Geometry check sheet. Reference: the model listing, model coordinates, mm. A direction names the side the tool comes from. Round coordinates to 2 decimals unless told otherwise and drop trailing zeros. Order: outer loops, then holes, each group sorted by start corner. A loop starts at its lowest first (then second) coordinate and runs counter-clockwise, first axis right, second up. Notation, with made-up numbers: (74, 72.5) - (101, 72.5) arc R15 cw to (101, 83.5) - close; hole circle Ø10 at (-19, 36). An arc over 180 degrees is marked (long way). One line per question, with ' | ' between items. Start each with the question number.
Q1. Gauge pin test, flat ends, axial feed: P1, Ø5, axis at x = 1016, z = 9.5, coming from the -Y side; P2, Ø5.5, axis at x = 620.64, y = 525.38, coming from the +Z side; P3, Ø2, axis at y = -198.5, z = 8.5, coming from the -X side; P4, Ø1, axis at x = 1180.5, z = 14, coming from the -Y side. Record the tip position at first contact, or that the pin passes through.
Q2. Sectioned sample at A-A, the plane x = 1039.5. Enter the section's corners in (y, z) (3 decimals), then the cut area to 3 significant figures.
Q3. Mould release check, pull along Y, two halves, no side actions. Record for faces 1 (the face through (1024.915, 215.072, 9.392)), 2 (the face through (916.535, 592.185, 9.392)), 3 (the face through (653.954, 499.757, 9.392)): +Y half, -Y half, draft (parallel to the pull), parting line (faces both ways), or undercut.
Q4. Material ranges on line 1 along Y through (x, z) = (1060, 1.75); line 2 along Y through (x, z) = (1069.5, 7.75); line 3 along X through (y, z) = (219, 13.75), recorded low to high.
Q5. Sectioned sample at C-C, the plane z = 4. Give the number of separate pieces and of enclosed holes in the cut face, then the cut area to 3 significant figures.
Q6. Tool access check on faces 4 (the face through (960.42, 143.22, 9.39)), 5 (the face through (982.65, -163.13, 9.39)), 6 (the face through (989.135, -122.216, 4.696)). Record the directions out of +Z, -Z, +X, -X, +Y, -Y that give a thin tool (end or side, any length) a straight path to the whole face; none if there is none.
Q7. Sectioned sample at B-B, the plane y = -16. Enter the section's corners in (x, z), then the cut area to 3 significant figures.
```python
from build123d import *

# Parameters (mm, degrees)
F1_DEPTH = 19.05
F3_DEPTH = 9.525
F5_DEPTH = 9.525
F6_W     = 94.742
F6_H     = 19.05
F6_H_2   = 22.0252738774
F7_DEPTH = 19.558
F8_R     = 3.302
F9_DEPTH = 19.051


# Not quite as in the source:
# - ends of sketch curves that miss each other by under 0.0002 mm in the source are joined
# - a feature names something its author has since deleted; it is built from what else it names
# - the program builds the solid bodies; features that only make, move or delete a surface that nothing else refers to are left out


with BuildPart() as f1:
    # F0 (on Top) → F1 (new body)
    with BuildSketch(Plane.XY):
        with BuildLine():
            Line((727.2677384075, 507.6293858847), (727.2677384075, -289.3185215378))
            ThreePointArc((727.2677384075, -289.3185215378), (771.8616098047, -333.912392935), (816.4554812019, -289.3185215378))
            Line((816.4554812019, -289.3185215378), (816.4554812019, -221.6290421598))
            Line((816.4554812019, -221.6290421598), (1153.5588304871, -102.9697649078))
            Line((1153.5588304871, -102.9697649078), (1192.9737952894, -152.2336658633))
            ThreePointArc((1192.9737952894, -152.2336658633), (1256.5580507142, -165.3785793409), (1281.2649482254, -105.3342998163))
            Line((1281.2649482254, -105.3342998163), (881.6774022659, 394.10141923))
            ThreePointArc((881.6774022659, 394.10141923), (879.6100790274, 397.83144491), (878.8940586752, 402.0355181492))
            Line((878.8940586752, 402.0355181492), (878.8940586752, 569.9420720746))
            ThreePointArc((878.8940586752, 569.9420720746), (881.2296299338, 577.2815963686), (887.3773054254, 581.9215959395))
            Line((887.3773054254, 581.9215959395), (946.5202680448, 602.7397254948))
            Line((946.5202680448, 602.7397254948), (904.3527355464, 722.5349641439))
            Line((904.3527355464, 722.5349641439), (884.020881133, 715.3782178375))
            Line((884.020881133, 715.3782178375), (880.8583161956, 724.3628607361))
            Line((880.8583161956, 724.3628607361), (549.7442765695, 607.8118009104))
            Line((549.7442765695, 607.8118009104), (552.906841507, 598.8271580117))
            Line((552.906841507, 598.8271580117), (544.9670195991, 596.0323666485))
            Line((544.9670195991, 596.0323666485), (582.9177988478, 488.2166518643))
            ThreePointArc((582.9177988478, 488.2166518643), (589.40821497, 480.9809077363), (599.1140759625, 480.4538812492))
            Line((599.1140759625, 480.4538812492), (710.3509851577, 519.6089097496))
            ThreePointArc((710.3509851577, 519.6089097497), (721.9072627016, 517.9938146262), (727.2677384075, 507.6293858847))
        make_face()
        with BuildLine():
            ThreePointArc((844.5095176323, -110.7755588107), (829.4863568252, -108.6759351502), (822.5177384075, -95.2021777863))
            Line((822.5177384075, -95.2021777863), (822.5177384075, 279.3762959499))
            ThreePointArc((822.5177384075, 279.3762959499), (831.0136651683, 291.3602755977), (845.1343948168, 287.3103948691))
            Line((845.1343948168, 287.3103948691), (1078.976974464, -4.9643221252))
            ThreePointArc((1078.976974464, -4.9643221252), (1081.9579117622, -19.8218837855), (1071.5671003568, -30.8520317446))
            Line((1071.5671003568, -30.8520317446), (844.5095176323, -110.7755588107))
        make_face(mode=Mode.SUBTRACT)
        with BuildLine():
            Line((822.1982316908, 418.0308171084), (817.981478441, 430.0103409733))
            ThreePointArc((817.981478441, 430.0103409733), (804.7653209472, 436.3447634256), (798.4309001253, 423.1286012999))
            Line((798.4309001253, 423.1286012999), (802.6476533752, 411.149077435))
            Line((802.6476533752, 411.149077435), (787.6732485441, 405.8781358727))
            Line((787.6732485441, 405.8781358727), (783.4564952942, 417.8576597376))
            ThreePointArc((783.4564952942, 417.8576597376), (799.4943781806, 451.3191657439), (832.9558841868, 435.2812828576))
            Line((832.9558841868, 435.2812828576), (837.1726374367, 423.3017589927))
            Line((837.1726374367, 423.3017589927), (822.1982316908, 418.0308171084))
        make_face(mode=Mode.SUBTRACT)
    extrude(amount=F1_DEPTH)

    # F2 (on face) → F3 (cut)
    with BuildSketch(Plane.XY):
        with BuildLine():
            ThreePointArc((844.1222933391, -166.9052020902), (847.3560158569, -170.6500208272), (852.2954479263, -170.9374917442))
            Line((852.2954479263, -170.9374917442), (1129.8610507564, -72.1108335167))
            ThreePointArc((1129.8610507564, -72.1108335167), (1133.425786756, -68.9382065458), (1133.77435322, -64.1788572139))
            Line((1133.77435322, -64.1788572139), (1131.667577719, -57.6492424267))
            ThreePointArc((1131.667577719, -57.6492424267), (1128.4338552012, -53.9044236898), (1123.4944231318, -53.6169527728))
            Line((1123.4944231318, -53.6169527728), (845.9288203018, -152.4436110002))
            ThreePointArc((845.9288203018, -152.4436110002), (842.3640843021, -155.6162379711), (842.0155178382, -160.3755873031))
            Line((842.0155178382, -160.3755873031), (844.1222933391, -166.9052020902))
        make_face()
    extrude(amount=F3_DEPTH, mode=Mode.SUBTRACT)

    # F4 (on face) → F5 (cut)
    with BuildSketch(Plane.XY):
        Polygon((579.9443241227, 521.366756094), (586.5044770697, 502.9417796404), (921.8787370541, 622.3506942479), (916.3315891482, 637.930524532), (912.1286802343, 636.4340924814), (884.020881133, 715.3782178375), (880.8583161956, 724.3628607361), (862.3802941818, 717.9536434315), (892.7236092325, 632.7308033777), align=None)
    extrude(amount=F5_DEPTH, mode=Mode.SUBTRACT)

    # F6 (on face) → F7 (cut)
    with BuildSketch(Plane(origin=(729.8159568657, 583.9097126711, 0), x_dir=(-0.6247321984, 0.7808390873, 0), z_dir=(0.7808390873, 0.6247321984, 0))):
        with Locations((-357.8801403508, 9.525)):
            Rectangle(F6_W, F6_H)
        with Locations((-584.9891603508, 10.3152221296)):
            Rectangle(F6_W, F6_H_2)
    extrude(amount=-F7_DEPTH, mode=Mode.SUBTRACT)

    # F8 (on face) → F9 (cut, through all)
    with BuildSketch(Plane.XY):
        with BuildLine():
            ThreePointArc((902.3498094673, 663.8992240234), (899.5515171423, 659.5044786379), (904.4975380125, 657.8670707804))
            Line((904.4975380125, 657.8670707804), (902.3498094673, 663.8992240234))
        make_face()
        with BuildLine():
            ThreePointArc((887.5764301967, 705.3920317976), (884.8076232072, 701.0002222812), (889.7289379426, 699.3464555963))
            Line((889.7289379426, 699.3464555963), (887.5764301967, 705.3920317976))
        make_face()
        with BuildLine():
            Line((887.5764301967, 705.3920317976), (889.7289379426, 699.3464555963))
            ThreePointArc((889.7289379426, 699.3464555963), (890.8236579238, 700.5386106967), (891.2203335175, 702.107780571))
            ThreePointArc((891.2203335175, 702.107780571), (890.1290165833, 704.5605513272), (887.5764301967, 705.3920317976))
        make_face()
        with BuildLine():
            Line((902.3498094673, 663.8992240234), (904.4975380125, 657.8670707804))
            ThreePointArc((904.4975380125, 657.8670707804), (905.5745632393, 659.0559185948), (905.9642274527, 660.6120369276))
            ThreePointArc((905.9642274527, 660.6120369276), (904.8838934731, 663.0548639976), (902.3498094673, 663.8992240234))
        make_face()
        with Locations((880.5389518172, 617.9122097817)):
            Circle(F8_R)
        with BuildLine():
            ThreePointArc((623.7483495144, 526.4827509324), (617.3838130375, 524.8132146381), (623.9396392041, 525.3751926427))
            ThreePointArc((623.9396392041, 525.3751926427), (623.8914653707, 525.9371706472), (623.7483495144, 526.4827509324))
        make_face()
        with BuildLine():
            ThreePointArc((756.0284718398, 572.4049919407), (752.1644938352, 575.6588181073), (749.6157615295, 571.2974336509))
            ThreePointArc((749.6157615295, 571.2974336509), (753.2884498444, 569.1511657741), (756.0284718398, 572.4049919407))
        make_face()
        with Locations((1055.4790926394, -88.2571151612)):
            Circle(F8_R)
        with Locations((913.5925848765, -138.7755124943)):
            Circle(F8_R)
    extrude(amount=F9_DEPTH, mode=Mode.SUBTRACT)


solid = f1.part
```
Determined:
1) P1: stops at y = -152.27 | P2: passes through | P3: stops at x = 727.27 | P4: stops at y = -137.27
2) outline: (-143.118, 0) - (-104.284, 0) - (-104.284, 9.525) - (-83.523, 9.525) - (-83.523, 0) - (-42.14, 0) - (-42.14, 19.05) - (-143.118, 19.05) - close; (44.377, 0) - (196.842, 0) - (196.842, 19.05) - (44.377, 19.05) - close | area: 4,630 mm2
3) face 1: +Y half | face 2: undercut | face 3: -Y half
4) line 1: y = -135.9 to -96.98, -76.22 to -34.92, 18.75 to 139.91, 159.57 to 171.22 | line 2: y = -132.56 to -93.6, -72.84 to -31.58, 6.88 to 128.04 | line 3: x = 727.27 to 822.52, 899.79 to 1021.77
5) separate pieces: 1 | enclosed holes: 3 | area: 219,000 mm2
6) face 4: +Z, -Z | face 5: +Z, -Z, -Y | face 6: -Z
7) outline: (727.27, 0) - (822.52, 0) - (822.52, 19.05) - (727.27, 19.05) - close; (1082.58, 0) - (1209.79, 0) - (1209.79, 19.05) - (1082.58, 19.05) - close | area: 4,240 mm2
